Source: CAD feature listing. Evaluate the final solid. Frame: model axes, mm. A direction names the side the tool comes from. Coordinates: 2 decimals unless noted, no trailing zeros. Order: outer loops, then holes, each group sorted by start corner. A loop starts at its lowest first (then second) coordinate and runs counter-clockwise, first axis right, second up.
```python
from build123d import *

# Parameters (mm, degrees)
SKETCH1_W           = 140
SKETCH1_H           = 200
BOSS_EXTRUDE1_DEPTH = 6
FILLET1_R           = 10
FILLET2_R           = 10
CHAMFER4_SIZE       = 5
CUT_EXTRUDE1_DEPTH  = 2
SKETCH7_R           = 3
CUT_EXTRUDE3_DEPTH  = 10
SKETCH8_R           = 4.5
CUT_EXTRUDE4_DEPTH  = 5


with BuildPart() as part:
    # Sketch1 → Boss-Extrude1 (new body)
    with BuildSketch(Plane(origin=(0, 0, 0), x_dir=(1, 0, 0), z_dir=(0, 1, 0))):
        with Locations((70, 100)):
            Rectangle(SKETCH1_W, SKETCH1_H)
        Polygon((10, 190), (50, 190), (60, 180), (80, 180), (90, 190), (130, 190), (130, 150), (110, 130), (110, 70), (130, 50), (130, 10), (90, 10), (80, 20), (60, 20), (50, 10), (10, 10), (10, 50), (30, 70), (30, 130), (10, 150), align=None, mode=Mode.SUBTRACT)
    extrude(amount=BOSS_EXTRUDE1_DEPTH)

    # Fillet1
    fillet1_edges = [part.edges().sort_by_distance(p)[0] for p in [
        (10, 3, -190),
    ]]
    fillet(fillet1_edges, radius=FILLET1_R)

    # Fillet2
    fillet2_edges = [part.edges().sort_by_distance(p)[0] for p in [
        (10, 3, -150),
        (30, 3, -130),
        (30, 3, -70),
        (10, 3, -50),
        (10, 3, -10),
        (50, 3, -10),
        (60, 3, -20),
        (80, 3, -20),
        (90, 3, -10),
        (130, 3, -10),
        (130, 3, -50),
        (110, 3, -70),
        (110, 3, -130),
        (130, 3, -150),
        (130, 3, -190),
        (90, 3, -190),
        (80, 3, -180),
        (60, 3, -180),
        (50, 3, -190),
    ]]
    fillet(fillet2_edges, radius=FILLET2_R)

    # Chamfer4
    chamfer4_edges = [part.edges().sort_by_distance(p)[0] for p in [
        (79.6846987, 0, -19.238795325),
        (60.3153013, 0, -19.238795325),
        (29.238795325, 0, -70.3153013),
        (29.238795325, 0, -129.6846987),
        (10.761204675, 0, -150.3153013),
        (10.761204675, 0, -49.6846987),
        (12.928932188, 0, -12.928932188),
        (49.6846987, 0, -10.761204675),
        (90.3153013, 0, -10.761204675),
        (127.071067812, 0, -12.928932188),
        (129.238795325, 0, -49.6846987),
        (129.238795325, 0, -150.3153013),
        (127.071067812, 0, -187.071067812),
        (90.3153013, 0, -189.238795325),
        (49.6846987, 0, -189.238795325),
        (10, 0, -167.071067812),
        (12.928932188, 0, -187.071067812),
        (20, 0, -140),
        (32.928932188, 0, -190),
        (30, 0, -100),
        (20, 0, -60),
        (10, 0, -32.928932188),
        (32.928932188, 0, -10),
        (55, 0, -15),
        (70, 0, -20),
        (85, 0, -15),
        (107.071067812, 0, -10),
        (130, 0, -32.928932188),
        (120, 0, -60),
        (110, 0, -100),
        (120, 0, -140),
        (130, 0, -167.071067812),
        (107.071067812, 0, -190),
        (85, 0, -185),
        (70, 0, -180),
        (55, 0, -185),
        (60.3153013, 0, -180.761204675),
        (79.6846987, 0, -180.761204675),
        (110.761204675, 0, -129.6846987),
        (110.761204675, 0, -70.3153013),
    ]]
    chamfer(chamfer4_edges, length=CHAMFER4_SIZE)

    # Sketch6 → Cut-Extrude1 (cut)
    with BuildSketch(Plane.XZ):
        with BuildLine():
            Line((118, -125), (118, -75))
            ThreePointArc((118, -75), (121, -72), (124, -75))
            Line((124, -75), (124, -125))
            ThreePointArc((124, -125), (121, -128), (118, -125))
        make_face()
        with BuildLine():
            Line((129, -133.028561836), (129, -67.028561836))
            ThreePointArc((129, -67.028561836), (132, -64.028561836), (135, -67.028561836))
            Line((135, -67.028561836), (135, -133.028561836))
            ThreePointArc((135, -133.028561836), (132, -136.028561836), (129, -133.028561836))
        make_face()
        with BuildLine():
            Line((22, -125), (22, -75))
            ThreePointArc((22, -75), (19, -72), (16, -75))
            Line((16, -75), (16, -125))
            ThreePointArc((16, -125), (19, -128), (22, -125))
        make_face()
        with BuildLine():
            Line((11, -133.028561836), (11, -67.028561836))
            ThreePointArc((11, -67.028561836), (8, -64.028561836), (5, -67.028561836))
            Line((5, -67.028561836), (5, -133.028561836))
            ThreePointArc((5, -133.028561836), (8, -136.028561836), (11, -133.028561836))
        make_face()
    extrude(amount=-CUT_EXTRUDE1_DEPTH, mode=Mode.SUBTRACT)

    # Sketch7 → Cut-Extrude3 (cut)
    with BuildSketch(Plane(origin=(0, 6, 0), x_dir=(1, 0, 0), z_dir=(0, 1, 0))):
        with Locations(Location((70, 191.8, 0), (0, 0, 270))):
            Circle(SKETCH7_R)
        with Locations(Location((8.166074554, 133, 0), (0, 0, 270))):
            Circle(SKETCH7_R)
        with Locations(Location((70, 8.2, 0), (0, 0, 90))):
            Circle(SKETCH7_R)
        with Locations(Location((8.166074554, 67, 0), (0, 0, 258.632230209))):
            Circle(SKETCH7_R)
        with Locations(Location((131.833925446, 67, 0), (0, 0, 270))):
            Circle(SKETCH7_R)
        with Locations(Location((131.833925446, 133, 0), (0, 0, 199.153699919))):
            Circle(SKETCH7_R)
    extrude(amount=-CUT_EXTRUDE3_DEPTH, mode=Mode.SUBTRACT)

    # Sketch8 → Cut-Extrude4 (cut)
    with BuildSketch(Plane.XZ):
        with Locations(Location((70, -8.2, 0), (0, 0, 270))):
            Circle(SKETCH8_R)
        with Locations(Location((8, -67.028561836, 0), (0, 0, 270))):
            Circle(SKETCH8_R)
        with Locations(Location((132, -67.028561836, 0), (0, 0, 228.189685104))):
            Circle(SKETCH8_R)
        with Locations(Location((8, -132.971438164, 0), (0, 0, 131.810314896))):
            Circle(SKETCH8_R)
        with Locations(Location((70, -191.8, 0), (0, 0, 90))):
            Circle(SKETCH8_R)
        with Locations(Location((132, -132.971438164, 0), (0, 0, 270))):
            Circle(SKETCH8_R)
    extrude(amount=-CUT_EXTRUDE4_DEPTH, mode=Mode.SUBTRACT)


solid = part.part
```
Q1. Section query A-A on z = -41.5. Output: boundary loops of the cut face in (x, y).
Solutions:
outline: (0, 0) - (5, 0) - (10, 5) - (10, 6) - (0, 6) - close; (130, 5) - (135, 0) - (140, 0) - (140, 6) - (130, 6) - close
Q2. Section query C-C on z = -87.5. Output: boundary loops of the cut face in (x, y).
Solutions:
outline: (0, 0) - (5, 0) - (5, 2) - (11, 2) - (11, 0) - (16, 0) - (16, 2) - (22, 2) - (22, 0) - (25, 0) - (30, 5) - (30, 6) - (0, 6) - close; (110, 5) - (115, 0) - (118, 0) - (118, 2) - (124, 2) - (124, 0) - (129, 0) - (129, 2) - (135, 2) - (135, 0) - (140, 0) - (140, 6) - (110, 6) - close
Q3. Material intervals for line 1 along X through (y, z) = (1.8, -8.2); line 2 along X through (y, z) = (4.35, -159); line 3 along Z through (x, y) = (128, 0.55), sorted ascending.
Solutions:
line 1: x = 0 to 14.08, 51.77 to 65.5, 74.5 to 88.23, 125.92 to 140
line 2: x = 0 to 9.35, 130.65 to 140
line 3: z = -200 to -192.03, -141.71 to -135.03, -130.91 to -69.09, -64.97 to -58.29, -7.97 to 0
Q4. Pin query (flat end, axial travel): P1, Ø1.1, axis at y = 5.5, z = -168.5, coming from the -X side; P2, Ø5.5, axis at x = 132, z = -67.03, coming from the +Y side; P3, Ø8, axis at x = 8.17, z = -67, coming from the -Y side. Return the tip coordinate at first contact, or that it passes through.
Solutions:
P1: stops at x = 0
P2: passes through
P3: stops at y = 5
Q5. Set-up query: faces 1 (the flat face through (33, 3, -192)), 2 (the flat face through (85, 5.5, -15)), 3 (the flat face through (22, 6, -101)). Return all of +Z, -Z, +X, -X, +Y, -Y with unobstructed straight access to the full face (end or side cutting, diameter ignored); none if empty.
Solutions:
face 1: -Y
face 2: +Y, -Y
face 3: +Z, -Z, +X, -X, +Y
Q6. Pull-direction query (X, two-part tool) for faces 4 (the conical face through (128.51, 3.09, -188.33)), 5 (the flat face through (23, 0, -100)); classes: pulls with the +X half, pulls with the -X half, needs draft (parallel to the pull), parting line crosses it, or undercut.
Solutions:
face 4: undercut
face 5: needs draft
Q7. Section query B-B on x = 70. Output: boundary loops of the cut face in (y, z).
Solutions:
outline: (0, -200) - (6, -200) - (6, -194.8) - (5, -194.8) - (5, -196.3) - (0, -196.3) - close; (0, -187.3) - (5, -187.3) - (5, -188.8) - (6, -188.8) - (6, -180) - (5, -180) - (0, -185) - close; (0, -15) - (5, -20) - (6, -20) - (6, -11.2) - (5, -11.2) - (5, -12.7) - (0, -12.7) - close; (0, -3.7) - (5, -3.7) - (5, -5.2) - (6, -5.2) - (6, 0) - (0, 0) - close
